Build history of the part. All positions in model axes, mm. Face numbers are marked on the shaded views. Coordinates: 2 decimals unless noted, no trailing zeros. Write each loop counter-clockwise with the first axis right and the second up, starting at its lowest first coordinate (ties: lowest second). Pieces come first, ordered by that corner, then holes.
```python
from build123d import *

# Parameters (mm, degrees)
ESQUISSE1_R        = 3
ESQUISSE1_R_2      = 1.5
BOSS_EXTRU_1_DEPTH = 3
CONG_1_R           = 0.5


with BuildPart() as part:
    # Esquisse1 → Boss.-Extru.1 (new body)
    with BuildSketch(Plane.XY):
        with BuildLine():
            ThreePointArc((-9.967950619, 9.398353751), (-19.856771897, 10.843547876), (-19.255850538, 0.867763905))
            ThreePointArc((-19.255850538, 0.867763905), (-11.16183771, -4.367412674), (-2.599104383, -8.794569261))
            ThreePointArc((-2.599104383, -8.794569261), (0.527471635, -8.932442445), (2.869569032, -6.856613359))
            ThreePointArc((2.869569032, -6.856613359), (5.106974254, -5.597078916), (7.101036237, -7.214523181))
            ThreePointArc((7.101036237, -7.214523181), (7.91789358, -9.198392931), (9.106885228, -10.984252378))
            ThreePointArc((9.106885228, -10.984252378), (12.345329643, -13.241699917), (16.286687996, -13.463704315))
            ThreePointArc((16.286687996, -13.463704315), (18.195594291, -14.034021941), (18.707504902, -15.959413581))
            ThreePointArc((18.707504902, -15.959413581), (25.123132348, -7.73541187), (19.778982477, 1.22196173))
            ThreePointArc((19.778982477, 1.22196173), (10.927169302, 5.05077079), (1.899061951, 8.443063964))
            ThreePointArc((1.899061951, 8.443063964), (-1.768338506, 8.299023868), (-4.357336538, 5.697550659))
            ThreePointArc((-4.357336538, 5.697550659), (-6.576456411, 4.361139029), (-8.561108443, 6.025964956))
            ThreePointArc((-8.561108443, 6.025964956), (-9.144248361, 7.762336434), (-9.967950619, 9.398353751))
        make_face()
        Circle(ESQUISSE1_R, mode=Mode.SUBTRACT)
        with Locations((-15.5, 6.1)):
            Circle(ESQUISSE1_R_2, mode=Mode.SUBTRACT)
        with Locations((13.7, -6.9)):
            Circle(ESQUISSE1_R_2, mode=Mode.SUBTRACT)
        with Locations((21.53, -9.653379741)):
            Circle(ESQUISSE1_R_2, mode=Mode.SUBTRACT)
    extrude(amount=BOSS_EXTRU_1_DEPTH)

    # Congé1
    cong_1_edges = [part.edges().sort_by_distance(p)[0] for p in [
        (18.707504902, -15.959413581, 1.5),
    ]]
    fillet(cong_1_edges, radius=CONG_1_R)


solid = part.part
```
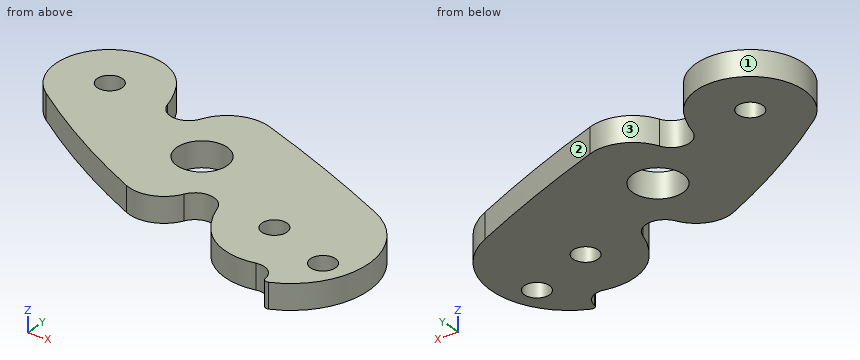
1. Saw through at A-A on x = 13.7. List the corners of the cut face in (y, z).
Computed values:
outline: (-13.57, 0) - (-8.4, 0) - (-8.4, 3) - (-13.57, 3) - close; (-5.4, 0) - (3.91, 0) - (3.91, 3) - (-5.4, 3) - close
2. Saw through at C-C on x = -11.5. List the corners of the cut face in (y, z), plus the area to 3 significant figures.
Computed values:
outline: (-4.17, 0) - (11.15, 0) - (11.15, 3) - (-4.17, 3) - close
area: 46.0 mm2
3. Flat gauge pins, fed straight in: pin 1 (12 mm diameter, centred on x = -2, y = 4, fed in from -Z); pin 2 (5 mm diameter, centred on x = 4, y = -12, fed in from -Z). Where does each tip first touch, or does it go through?
Computed values:
pin 1: stops at z = 0
pin 2: passes through
4. Saw through at B-B on y = 0. List the corners of the cut face in (x, z).
Computed values:
outline: (-18.03, 0) - (-3, 0) - (-3, 3) - (-18.03, 3) - close; (3, 0) - (21.74, 0) - (21.74, 3) - (3, 3) - close
5. Mould opens along X. For the marked faces 1, 2 and 3 say: +X half, -X half, draft (parallel to the pull), parting line (faces both ways), or undercut.
Computed values:
face 1: parting line
face 2: +X half
face 3: undercut
6. Saw through at D-D on z = 2.25. State how many separate pieces and enclosed holes the cut face has, plus the area to 3 significant figures.
Computed values:
separate pieces: 1
enclosed holes: 4
area: 623 mm2
7. Probe line 1 along X through (y, z) = (-10.75, 1.65); line 2 along Y through (x, z) = (21.53, 2.25) (3 decimals); line 3 along Y through (x, z) = (22, 1.95). List the from-to ranges inside material, lowest first.
Computed values:
line 1: x = 8.92 to 20.51, 22.55 to 24.41
line 2: y = -14.485 to -11.153, -8.153 to 0.164
line 3: y = -14.1 to -11.08, -8.23 to -0.22
